from build123d import *

# Parameters (mm, degrees)
BOSS_EXTRUDE1_DEPTH = 2
CUT_EXTRUDE1_REACH  = 44.755
SKETCH2_R           = 1.5
SKETCH3_W           = 1.5
SKETCH3_H           = 1.5
BOSS_EXTRUDE2_DEPTH = 2
SKETCH6_W           = 1.5
SKETCH6_H           = 1.17146139
BOSS_EXTRUDE5_DEPTH = 5
FILLET1_R           = 0.2
BOSS_EXTRUDE6_DEPTH = 0.3


with BuildPart() as part:
    # Sketch1 → Boss-Extrude1 (new body)
    with BuildSketch(Plane.XY):
        with BuildLine():
            Line((-31.956856316, -21.666666667), (-31.956856316, 26.333333333))
            ThreePointArc((-31.956856316, 26.333333333), (-31.371069879, 27.747546896), (-29.956856316, 28.333333333))
            Line((-29.956856316, 28.333333333), (-8.956856316, 28.333333333))
            ThreePointArc((-8.956856316, 28.333333333), (-7.542642754, 27.747546896), (-6.956856316, 26.333333333))
            Line((-6.956856316, 26.333333333), (-6.956856316, -21.666666667))
            Line((-6.956856316, -21.666666667), (-10.956856316, -26.666666667))
            Line((-10.956856316, -26.666666667), (-14.956856316, -21.666666667))
            Line((-14.956856316, -21.666666667), (-14.956856316, 16.627941441))
            ThreePointArc((-14.956856316, 16.627941441), (-19.456856316, 20.722627268), (-23.956856316, 16.627941441))
            Line((-23.956856316, 16.627941441), (-23.956856316, -21.666666667))
            Line((-23.956856316, -21.666666667), (-27.956856316, -26.666666667))
            Line((-27.956856316, -26.666666667), (-31.956856316, -21.666666667))
        make_face()
    extrude(amount=BOSS_EXTRUDE1_DEPTH)

    # Sketch2 → Cut-Extrude1 (cut, up to next)
    with BuildSketch(Plane(origin=(0, 0, 0), x_dir=(-1, 0, 0), z_dir=(0, 0, -1)), mode=Mode.PRIVATE) as cut_extrude1_sk1:
        with Locations((8.956856316, 26.146893442)):
            Circle(SKETCH2_R)
    cut_extrude1_tool1 = extrude(cut_extrude1_sk1.sketch, amount=-CUT_EXTRUDE1_REACH, mode=Mode.PRIVATE) & part.part
    # Sketch2 → Cut-Extrude1 (cut, up to next)
    with BuildSketch(Plane(origin=(0, 0, 0), x_dir=(-1, 0, 0), z_dir=(0, 0, -1)), mode=Mode.PRIVATE) as cut_extrude1_sk2:
        with Locations((29.956856316, 26.146893442)):
            Circle(SKETCH2_R)
    cut_extrude1_tool2 = extrude(cut_extrude1_sk2.sketch, amount=-CUT_EXTRUDE1_REACH, mode=Mode.PRIVATE) & part.part
    add(cut_extrude1_tool1.solids().sort_by_distance((-8.956856, 26.146893, 0))[0], mode=Mode.SUBTRACT)
    add(cut_extrude1_tool2.solids().sort_by_distance((-29.956856, 26.146893, 0))[0], mode=Mode.SUBTRACT)

    # Sketch3 → Boss-Extrude2 (add)
    with BuildSketch(Plane(origin=(0, 0, 0), x_dir=(-1, 0, 0), z_dir=(0, 0, -1))):
        with Locations((20.175136294, 26.788088759)):
            Rectangle(SKETCH3_W, SKETCH3_H)
        with Locations((18.175136294, 26.788088759)):
            Rectangle(SKETCH3_W, SKETCH3_H)
    extrude(amount=BOSS_EXTRUDE2_DEPTH)

    # Sketch6 → Boss-Extrude5 (add)
    with BuildSketch(Plane(origin=(0, 27.538088759, 0), x_dir=(1, 0, 0), z_dir=(0, 1, 0))):
        with Locations((-18.175136294, 1.414269305)):
            Rectangle(SKETCH6_W, SKETCH6_H)
        with Locations((-20.175136294, 1.414269305)):
            Rectangle(SKETCH6_W, SKETCH6_H)
    extrude(amount=BOSS_EXTRUDE5_DEPTH)

    # Fillet1
    fillet1_edges = [part.edges().sort_by_distance(p)[0] for p in [
        (-18.175136294, 26.038088759, -2),
        (-20.175136294, 26.038088759, -2),
    ]]
    fillet(fillet1_edges, radius=FILLET1_R)

    # Sketch7 → Boss-Extrude6 (add)
    with BuildSketch(Plane(origin=(0, 0, 0), x_dir=(-1, 0, 0), z_dir=(0, 0, -1))):
        with BuildLine():
            Line((8.956856316, 16.860436634), (8.956856316, 15.572285455))
            Line((8.956856316, 15.572285455), (7.994072914, 15.572285455))
            ThreePointArc((7.994072914, 15.572285455), (7.553465888, 14.508565999), (7.994072914, 13.444846543))
            Line((7.994072914, 13.444846543), (8.956856316, 13.444846543))
            Line((8.956856316, 13.444846543), (8.956856316, 9.572285455))
            Line((8.956856316, 9.572285455), (7.994072914, 9.572285455))
            ThreePointArc((7.994072914, 9.572285455), (7.553465888, 8.508565999), (7.994072914, 7.444846543))
            Line((7.994072914, 7.444846543), (8.956856316, 7.444846543))
            Line((8.956856316, 7.444846543), (8.956856316, 3.572285455))
            Line((8.956856316, 3.572285455), (7.994072914, 3.572285455))
            ThreePointArc((7.994072914, 3.572285455), (7.553465888, 2.508565999), (7.994072914, 1.444846543))
            Line((7.994072914, 1.444846543), (8.956856316, 1.444846543))
            Line((8.956856316, 1.444846543), (8.956856316, -2.427714545))
            Line((8.956856316, -2.427714545), (7.994072914, -2.427714545))
            ThreePointArc((7.994072914, -2.427714545), (7.553465888, -3.491434001), (7.994072914, -4.555153457))
            Line((7.994072914, -4.555153457), (8.956856316, -4.555153457))
            Line((8.956856316, -4.555153457), (8.956856316, -8.427714545))
            Line((8.956856316, -8.427714545), (7.994072914, -8.427714545))
            ThreePointArc((7.994072914, -8.427714545), (7.553465888, -9.491434001), (7.994072914, -10.555153457))
            Line((7.994072914, -10.555153457), (8.956856316, -10.555153457))
            Line((8.956856316, -10.555153457), (8.956856316, -14.427714545))
            Line((8.956856316, -14.427714545), (7.994072914, -14.427714545))
            ThreePointArc((7.994072914, -14.427714545), (7.553465888, -15.491434001), (7.994072914, -16.555153457))
            Line((7.994072914, -16.555153457), (8.956856316, -16.555153457))
            Line((8.956856316, -16.555153457), (8.956856316, -19.220690879))
            ThreePointArc((8.956856316, -19.220690879), (10.956856316, -21.220690879), (12.956856316, -19.220690879))
            Line((12.956856316, -19.220690879), (12.956856316, -16.555153457))
            Line((12.956856316, -16.555153457), (13.997034927, -16.555153457))
            ThreePointArc((13.997034927, -16.555153457), (14.437641952, -15.491434001), (13.997034927, -14.427714545))
            Line((13.997034927, -14.427714545), (12.956856316, -14.427714545))
            Line((12.956856316, -14.427714545), (12.956856316, -10.555153457))
            Line((12.956856316, -10.555153457), (13.997034927, -10.555153457))
            ThreePointArc((13.997034927, -10.555153457), (14.437641952, -9.491434001), (13.997034927, -8.427714545))
            Line((13.997034927, -8.427714545), (12.956856316, -8.427714545))
            Line((12.956856316, -8.427714545), (12.956856316, -4.555153457))
            Line((12.956856316, -4.555153457), (13.997034927, -4.555153457))
            ThreePointArc((13.997034927, -4.555153457), (14.437641952, -3.491434001), (13.997034927, -2.427714545))
            Line((13.997034927, -2.427714545), (12.956856316, -2.427714545))
            Line((12.956856316, -2.427714545), (12.956856316, 1.444846543))
            Line((12.956856316, 1.444846543), (13.997034927, 1.444846543))
            ThreePointArc((13.997034927, 1.444846543), (14.437641952, 2.508565999), (13.997034927, 3.572285455))
            Line((13.997034927, 3.572285455), (12.956856316, 3.572285455))
            Line((12.956856316, 3.572285455), (12.956856316, 7.444846543))
            Line((12.956856316, 7.444846543), (13.997034927, 7.444846543))
            ThreePointArc((13.997034927, 7.444846543), (14.437641952, 8.508565999), (13.997034927, 9.572285455))
            Line((13.997034927, 9.572285455), (12.956856316, 9.572285455))
            Line((12.956856316, 9.572285455), (12.956856316, 13.444846543))
            Line((12.956856316, 13.444846543), (13.997034927, 13.444846543))
            ThreePointArc((13.997034927, 13.444846543), (14.437641952, 14.508565999), (13.997034927, 15.572285455))
            Line((13.997034927, 15.572285455), (12.956856316, 15.572285455))
            Line((12.956856316, 15.572285455), (12.956856316, 16.860436634))
            Line((12.956856316, 16.860436634), (8.956856316, 16.860436634))
        make_face()
        with BuildLine():
            Line((30.997034927, -16.555153457), (29.956856316, -16.555153457))
            Line((29.956856316, -16.555153457), (29.956856316, -19.220690879))
            ThreePointArc((29.956856316, -19.220690879), (27.956856316, -21.220690879), (25.956856316, -19.220690879))
            Line((25.956856316, -19.220690879), (25.956856316, -16.555153457))
            Line((25.956856316, -16.555153457), (24.994072914, -16.555153457))
            ThreePointArc((24.994072914, -16.555153457), (24.553465888, -15.491434001), (24.994072914, -14.427714545))
            Line((24.994072914, -14.427714545), (25.956856316, -14.427714545))
            Line((25.956856316, -14.427714545), (25.956856316, -10.555153457))
            Line((25.956856316, -10.555153457), (24.994072914, -10.555153457))
            ThreePointArc((24.994072914, -10.555153457), (24.553465888, -9.491434001), (24.994072914, -8.427714545))
            Line((24.994072914, -8.427714545), (25.956856316, -8.427714545))
            Line((25.956856316, -8.427714545), (25.956856316, -4.555153457))
            Line((25.956856316, -4.555153457), (24.994072914, -4.555153457))
            ThreePointArc((24.994072914, -4.555153457), (24.553465888, -3.491434001), (24.994072914, -2.427714545))
            Line((24.994072914, -2.427714545), (25.956856316, -2.427714545))
            Line((25.956856316, -2.427714545), (25.956856316, 1.444846543))
            Line((25.956856316, 1.444846543), (24.994072914, 1.444846543))
            ThreePointArc((24.994072914, 1.444846543), (24.553465888, 2.508565999), (24.994072914, 3.572285455))
            Line((24.994072914, 3.572285455), (25.956856316, 3.572285455))
            Line((25.956856316, 3.572285455), (25.956856316, 7.444846543))
            Line((25.956856316, 7.444846543), (24.994072914, 7.444846543))
            ThreePointArc((24.994072914, 7.444846543), (24.553465888, 8.508565999), (24.994072914, 9.572285455))
            Line((24.994072914, 9.572285455), (25.956856316, 9.572285455))
            Line((25.956856316, 9.572285455), (25.956856316, 13.444846543))
            Line((25.956856316, 13.444846543), (24.994072914, 13.444846543))
            ThreePointArc((24.994072914, 13.444846543), (24.553465888, 14.508565999), (24.994072914, 15.572285455))
            Line((24.994072914, 15.572285455), (25.956856316, 15.572285455))
            Line((25.956856316, 15.572285455), (25.956856316, 16.860436634))
            Line((25.956856316, 16.860436634), (29.956856316, 16.860436634))
            Line((29.956856316, 16.860436634), (29.956856316, 15.572285455))
            Line((29.956856316, 15.572285455), (30.997034927, 15.572285455))
            ThreePointArc((30.997034927, 15.572285455), (31.437641952, 14.508565999), (30.997034927, 13.444846543))
            Line((30.997034927, 13.444846543), (29.956856316, 13.444846543))
            Line((29.956856316, 13.444846543), (29.956856316, 9.572285455))
            Line((29.956856316, 9.572285455), (30.997034927, 9.572285455))
            ThreePointArc((30.997034927, 9.572285455), (31.437641952, 8.508565999), (30.997034927, 7.444846543))
            Line((30.997034927, 7.444846543), (29.956856316, 7.444846543))
            Line((29.956856316, 7.444846543), (29.956856316, 3.572285455))
            Line((29.956856316, 3.572285455), (30.997034927, 3.572285455))
            ThreePointArc((30.997034927, 3.572285455), (31.437641952, 2.508565999), (30.997034927, 1.444846543))
            Line((30.997034927, 1.444846543), (29.956856316, 1.444846543))
            Line((29.956856316, 1.444846543), (29.956856316, -2.427714545))
            Line((29.956856316, -2.427714545), (30.997034927, -2.427714545))
            ThreePointArc((30.997034927, -2.427714545), (31.437641952, -3.491434001), (30.997034927, -4.555153457))
            Line((30.997034927, -4.555153457), (29.956856316, -4.555153457))
            Line((29.956856316, -4.555153457), (29.956856316, -8.427714545))
            Line((29.956856316, -8.427714545), (30.997034927, -8.427714545))
            ThreePointArc((30.997034927, -8.427714545), (31.437641952, -9.491434001), (30.997034927, -10.555153457))
            Line((30.997034927, -10.555153457), (29.956856316, -10.555153457))
            Line((29.956856316, -10.555153457), (29.956856316, -14.427714545))
            Line((29.956856316, -14.427714545), (30.997034927, -14.427714545))
            ThreePointArc((30.997034927, -14.427714545), (31.437641952, -15.491434001), (30.997034927, -16.555153457))
        make_face()
    extrude(amount=BOSS_EXTRUDE6_DEPTH)


solid = part.part
Could you check a few things on this model? Use its own coordinates, in mm. A direction names the side the tool comes from. Round coordinates to 2 decimals unless told otherwise and drop trailing zeros. Write each loop counter-clockwise with the first axis right and the second up, starting at its lowest first coordinate (ties: lowest second). Pieces come first, ordered by that corner, then holes. Notation, with made-up numbers: (29.5, 44.5) - (77.5, 44.5) arc R20 ccw to (77.5, 81.5) - close; hole circle Ø7 at (2, 3.25). An arc over 180 degrees is marked (long way). Use a Markdown table: item, result.
Q1. I want a section at A-A (y = -7.5). List the corners of the cut face in (x, z) for me.
Output values:
| item | result |
|---|---|
| outline | (-31.96, 0) - (-29.96, 0) - (-29.96, -0.3) - (-25.96, -0.3) - (-25.96, 0) - (-23.96, 0) - (-23.96, 2) - (-31.96, 2) - close; (-14.96, 0) - (-12.96, 0) - (-12.96, -0.3) - (-8.96, -0.3) - (-8.96, 0) - (-6.96, 0) - (-6.96, 2) - (-14.96, 2) - close |
Q2. I want a section at B-B (z = 1.25). List the corners of the cut face in (x, y) for me.
Output values:
| item | result |
|---|---|
| outline | (-31.96, -21.67) - (-27.96, -26.67) - (-23.96, -21.67) - (-23.96, 16.63) arc R4.52 cw to (-14.96, 16.63) - (-14.96, -21.67) - (-10.96, -26.67) - (-6.96, -21.67) - (-6.96, 26.33) arc R2 ccw to (-8.96, 28.33) - (-29.96, 28.33) arc R2 ccw to (-31.96, 26.33) - close; hole circle Ø3 at (-29.96, 26.15); hole circle Ø3 at (-8.96, 26.15) |
Q3. Thinking about a two-plate mould opening in X: for faces 1 (the cylindrical face through (-7.6, 27.8, 1)), 2 (the flat face through (-18, 26.038, -1)), 3 (the flat face through (-12.93, -24.2, 0.99)), which applies, released by +X, released by -X, zero draft, split by the parting line, or undercut?
Output values:
| item | result |
|---|---|
| face 1 | released by +X |
| face 2 | zero draft |
| face 3 | undercut |
Q4. Please list where these lines run through material, in increasing order: L1, parallel to X at y = -11.5, z = 0.15; L2, parallel to Z at x = -9.5, y = -13; L3, parallel to Z at x = -27, y = -24.
Output values:
| item | result |
|---|---|
| L1 | -31.96 to -23.96, -14.96 to -6.96 |
| L2 | -0.3 to 2 |
| L3 | 0 to 2 |
Q5. I want a section at D-D (y = -23). List the corners of the cut face in (x, z) for me, plus the area to 3 significant figures.
Output values:
| item | result |
|---|---|
| outline | (-30.89, 0) - (-25.02, 0) - (-25.02, 2) - (-30.89, 2) - close; (-13.89, 0) - (-8.02, 0) - (-8.02, 2) - (-13.89, 2) - close |
| area | 23.5 mm2 |
Q6. I want a section at C-C (x = -11.75). List the corners of the cut face in (y, z) for me.
Output values:
| item | result |
|---|---|
| outline | (-25.68, 0) - (-21.06, 0) - (-21.06, -0.3) - (16.86, -0.3) - (16.86, 0) - (28.33, 0) - (28.33, 2) - (-25.68, 2) - close |
Q7. For pin 1 (1.6 mm diameter, centred on x = -18, z = -1, fed in from -Y); pin 2 (1 mm diameter, centred on x = -11.5, y = -2, fed in from -Z), each with a flat end and sliding along its axis, tell me the tip position at first contact or that it passes through.
Output values:
| item | result |
|---|---|
| pin 1 | y = 26.04 |
| pin 2 | z = -0.3 |
Q8. For faces 4 (the flat face through (-17.425, 29, -1)), 5 (the flat face through (-20, 26.038, -1)), 6 (the flat face through (-14.957, -3, 1)), which set-ups out of +Z, -Z, +X, -X, +Y, -Y let a thin tool reach every point of the face, with its end or its side?
Output values:
| item | result |
|---|---|
| face 4 | -Z, +X, +Y, -Y |
| face 5 | -Z, +X, -X, -Y |
| face 6 | +Z, -Z, -Y |
